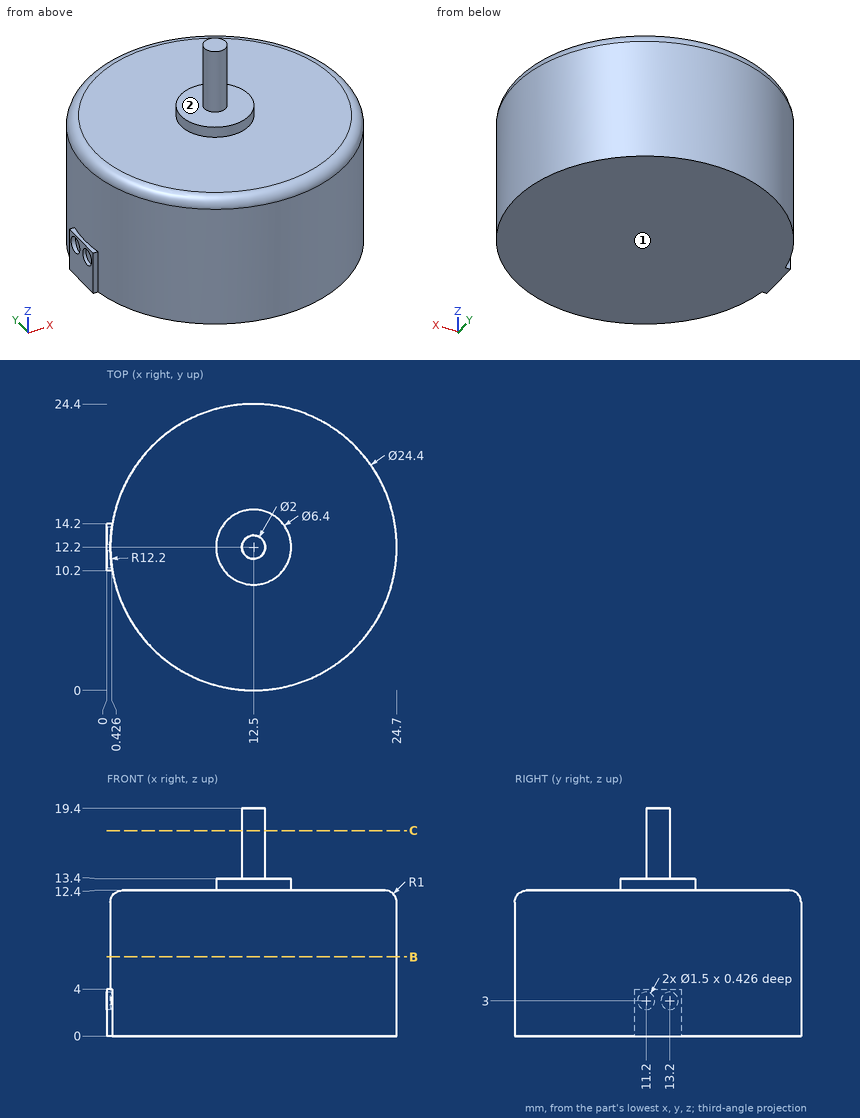
Could you check a few things on this drawing? It's one solid part, dimensions in mm from its lowest x, y, z. A direction names the side the tool comes from. Give positions to 0.01 mm unless a question says otherwise; leave off trailing zeros. Order: outer loops, then holes, each group sorted by start corner. A loop starts at its lowest first (then second) coordinate and runs counter-clockwise, first axis right, second up. Notation, with made-up numbers: M 1,-15 L 47,-15 A26 ccw 47,23 Z; hole C 51.5,80 d2. An arc over 180 degrees is marked long. Use one line per item in the form item = value.
Item 1: Will these pins go through, and if not, where does the flat tip stop? pin 1 Ø0.5 at (x, y) = (0, 13) entering from +Z; pin 2 Ø6 at (x, z) = (2.5, 11) entering from -Y; pin 3 Ø4 at (y, z) = (3.5, 14) entering from -X.
Values follow:
pin_1 = 4
pin_2 = 2.21
pin_3 = 3.67
Item 2: For the marked faces 1 and 2, which set-ups out of +Z, -Z, +X, -X, +Y, -Y let a thin tool reach every point of the face, with its end or its side?
Values follow:
face_1 = -Z, +X, -X, +Y, -Y
face_2 = +Z
Item 3: If I drill on line 1 along Y through (x, z) = (0.1, 3); line 2 along Z through (x, y) = (0.2, 13.2); line 3 along Z through (x, y) = (7.5, 20.25), over which ranges is the centre line in solid material (lowest first)? Write a range as [from, to].
Values follow:
line_1 = [10.2, 10.45], [11.95, 12.45], [13.95, 14.2]
line_2 = [0, 2.25], [3.75, 4]
line_3 = [0, 12.4]
Item 4: If we section it at B-B, the plane z = 6.75: Write out the boundary of the cut face in (x, y).
Values follow:
outline = C 12.5,12.2 d24.4
Item 5: If we section it at C-C, the plane z = 17.5: Write out the boundary of the cut face in (x, y).
Values follow:
outline = C 12.5,12.2 d2
